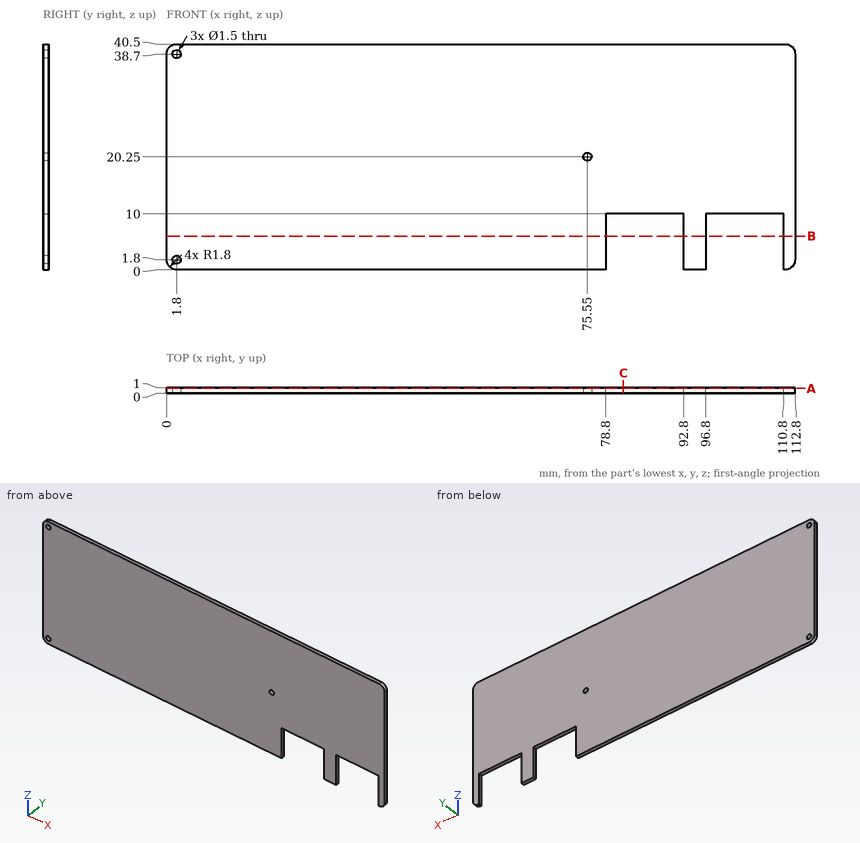
Design review of the part shown in the three views and the two pictorial views. Dimensions are in mm from the part's minimum x, y and z. Give positions to 0.01 mm unless a question says otherwise; leave off trailing zeros. Order: outer loops, then holes, each group sorted by start corner. A loop starts at its lowest first (then second) coordinate and runs counter-clockwise, first axis right, second up. Notation, with made-up numbers: M -30.75,24.5 L -7.75,24.5 A13 ccw -7.75,49.5 Z; hole C 42.25,81 d9. An arc over 180 degrees is marked long. Answer in a Markdown table with one row per item. Add a question column.
(1) For pin 1 (12 mm diameter, centred on x = 91, z = 19, fed in from -Y), flat-tipped, find the tip position at first contact; note if it passes through.
(2) Wall thickness on probe 1 along X at (y, z) = (0.5, 7.5); probe 2 along X at (y, z) = (0.7, 38.7); probe 3 along X at (y, z) = (0.45, 20.25): over which ranges is each line inside the solid? List them lowest first. Write a range as [from, to].
(3) Consider section B-B on z = 6. State the section outline as (x, y) points.
(4) Consider section C-C on x = 82. State the section outline as (y, z) points, and give its area (3 significant figures).
(5) Consider section A-A on y = 0.85. State the section outline as (x, z) points.
Evaluation:
| question | item | result |
|---|---|---|
| 1 | pin 1 | stops at y = 0 |
| 2 | probe 1 | x = [0, 78.8], [92.8, 96.8], [110.8, 112.8] |
| 2 | probe 2 | x = [0, 1.05], [2.55, 112.8] |
| 2 | probe 3 | x = [0, 74.8], [76.3, 112.8] |
| 3 | outline | M 0,0 L 78.8,0 L 78.8,1 L 0,1 Z; M 92.8,0 L 96.8,0 L 96.8,1 L 92.8,1 Z; M 110.8,0 L 112.8,0 L 112.8,1 L 110.8,1 Z |
| 4 | outline | M 0,10 L 1,10 L 1,40.5 L 0,40.5 Z |
| 4 | area | 30.5 mm^2 |
| 5 | outline | M 0,1.8 A1.8 ccw 1.8,0 L 78.8,0 L 78.8,10 L 92.8,10 L 92.8,0 L 96.8,0 L 96.8,10 L 110.8,10 L 110.8,0 L 111,0 A1.8 ccw 112.8,1.8 L 112.8,38.7 A1.8 ccw 111,40.5 L 1.8,40.5 A1.8 ccw 0,38.7 Z; hole C 1.8,1.8 d1.5; hole C 1.8,38.7 d1.5; hole C 75.55,20.25 d1.5 |
